Verification items for the finished model (mm, model axes). A direction names the side the tool comes from. Coordinates: 2 decimals unless noted, no trailing zeros. Write each loop counter-clockwise with the first axis right and the second up, starting at its lowest first coordinate (ties: lowest second). Pieces come first, ordered by that corner, then holes. Notation, with made-up numbers: (57, -16) -> (109, -16) arc R26 ccw to (109, -2) -> close; hole circle Ø9 at (72, 20). An arc over 180 degrees is marked (long way). Use CSV: the item, a comma, the result in double quotes.
```python
from build123d import *

# Parameters (mm, degrees)
BOSS_EXTRUDE1_DEPTH = 25.4
CUT_EXTRUDE1_DEPTH  = 5.08
SKETCH3_OUTSIDE_W   = 13.788
SKETCH3_OUTSIDE_H   = 14.77
SKETCH3_OUTSIDE_R   = 3.175
CUT_EXTRUDE2_DEPTH  = 13.7


with BuildPart() as part:
    # Sketch1 → Boss-Extrude1 (new body)
    with BuildSketch(Plane.XY):
        Polygon((0, 3.666174209), (-3.175, 1.833087105), (-3.175, -1.833087105), (0, -3.666174209), (3.175, -1.833087105), (3.175, 1.833087105), align=None)
    extrude(amount=-BOSS_EXTRUDE1_DEPTH)

    # Sketch2 → Cut-Extrude1 (cut)
    with BuildSketch(Plane.XY):
        with BuildLine():
            Line((-1.109862584, -0.6206744), (1.109862584, -0.6206744))
            ThreePointArc((1.109862584, -0.6206744), (0, 1.2716256), (-1.109862584, -0.6206744))
        make_face()
    extrude(amount=-CUT_EXTRUDE1_DEPTH, mode=Mode.SUBTRACT)

    # Sketch3 outside → Cut-Extrude2 (cut, through all)
    with BuildSketch(Plane.XY.offset(-12.7)):
        Rectangle(SKETCH3_OUTSIDE_W, SKETCH3_OUTSIDE_H)
        Circle(SKETCH3_OUTSIDE_R, mode=Mode.SUBTRACT)
    extrude(amount=-CUT_EXTRUDE2_DEPTH, mode=Mode.SUBTRACT)


solid = part.part
```
1) Cross-section at B-B (x = -2). Record the boundary of the cut face in (y, z), plus the area to 3 significant figures.
Return value:
outline,"(-2.51, -12.7) -> (-2.47, -12.7) -> (-2.47, -25.4) -> (2.47, -25.4) -> (2.47, -12.7) -> (2.51, -12.7) -> (2.51, 0) -> (-2.51, 0) -> close"
area,"126 mm2"
2) Cross-section at C-C (y = 0.25). Record the boundary of the cut face in (x, z) (3 decimals).
Return value:
outline,"(-3.175, -12.7) -> (-3.165, -12.7) -> (-3.165, -25.4) -> (3.165, -25.4) -> (3.165, -12.7) -> (3.175, -12.7) -> (3.175, 0) -> (1.247, 0) -> (1.247, -5.08) -> (-1.247, -5.08) -> (-1.247, 0) -> (-3.175, 0) -> close"
3) Mould release check, pull along X, two halves, no side actions. Record for faces 1 (the flat face through (-1.61, -2.737, -6.261)), 2 (the flat face through (0, 3.4, -12.7)), 3 (the flat face through (0, -0.621, -3)): released by +X, released by -X, zero draft, split by the parting line, or undercut.
Return value:
face 1,"released by -X"
face 2,"zero draft"
face 3,"undercut"
4) Scan lines: L1, parallel to X at y = 0, z = -3.4 (3 decimals); L2, parallel to Z at x = -0.5, y = 0.25; L3, parallel to X at y = 3, z = -7.5. Record each from-to range of solid material in increasing order.
Return value:
L1,"-3.175 to -1.272, 1.272 to 3.175"
L2,"-25.4 to -5.08"
L3,"-1.15 to 1.15"
5) Cross-section at A-A (z = -5.75). Record the boundary of the cut face in (x, y) (3 decimals).
Return value:
outline,"(-3.175, -1.833) -> (0, -3.666) -> (3.175, -1.833) -> (3.175, 1.833) -> (0, 3.666) -> (-3.175, 1.833) -> close"
6) Cross-section at D-D (y = 2.25). Record the boundary of the cut face in (x, z), plus the area to 3 significant figures.
Return value:
outline,"(-2.45, -12.7) -> (-2.24, -12.7) -> (-2.24, -25.4) -> (2.24, -25.4) -> (2.24, -12.7) -> (2.45, -12.7) -> (2.45, 0) -> (-2.45, 0) -> close"
area,"119 mm2"
7) Set-up check for faces 4 (the flat face through (2.9, 1.7, -12.7)), 5 (the flat face through (0, 0, -5.08)), 6 (the flat face through (-0.01, -3.34, -12.7)), 7 (the flat face through (2.9, -1.7, -12.7)): record each of +Z, -Z, +X, -X, +Y, -Y from which the full face is reachable in a straight line by a thin tool's end or side.
Return value:
face 4,"-Z, +X, +Y"
face 5,"+Z"
face 6,"-Z, -Y"
face 7,"-Z, +X, -Y"
8) Gauge pin test, flat end, axial feed: pin 1 (1.5 mm diameter, centred on x = 1.5, z = -9, fed in from -Y). Record the tip position at first contact, or that the pin passes through.
Return value:
pin 1,"y = -3.23"
